Design review of the part built by this model. Coordinates are the model's own, in mm. A direction names the side the tool comes from. Coordinates: 2 decimals unless noted, no trailing zeros. Loops run counter-clockwise (first coordinate to the right, second up) from the corner with the lowest first, then second, coordinate; pieces in that order, holes last. Notation, with made-up numbers: (81.25, -20.5) -> (89.25, -20.5) arc R24 cw to (89.25, 1.5) -> close; hole circle Ø10 at (59, 26.25). An arc over 180 degrees is marked (long way). One line per item, written item: value. Start each with the question number.
1. Add section C-C on x = 22.5. Write out the cut boundary in (y, z), plus the area to 3 significant figures.
2. Add section B-B on z = 24.5. Write out the cut boundary in (x, y), plus the area to 3 significant figures.
3. Add section D-D on y = 19.5. Write out the cut boundary in (x, z).
4. Add section A-A on y = 34. Write out the cut boundary in (x, z), plus the area to 3 significant figures.
5. For probe 1 along X at (y, z) = (19, 21); probe 2 along Y at (x, z) = (23, 30); probe 3 along Y at (x, z) = (23, 28), list the stretches that pass through material, from the lowest coordinate up.
6. Machinability: for faces 1 (the flat face through (6, 35, 0)), 2 (the flat face through (0, 15, 16)), 3 (the flat face through (12.7, 15, 16)), which of the approach directions +Z, -Z, +X, -X, +Y, -Y give a long, thin tool a straight path to every point of the face, cutting with its end or side? Answer none if there is none.
7. Insertion check: pin 1 (3 mm diameter, centred on x = -2, z = 25.5, fed in from -Y); pin 2 (9.5 mm diameter, centred on y = 18.5, z = 20, fed in from +X). Each pin has a flat end and moves straight along its axis. Give the tip position at first contact, or say it passes through.
```python
from build123d import *

# Parameters (mm, degrees)
F1_DEPTH = 31.75
F3_DEPTH = 12.7
F5_DEPTH = 12.7


with BuildPart() as f1:
    # F0 (on Top) → F1 (new body)
    with BuildSketch(Plane.XY):
        Polygon((0, 25.4), (0, 0), (12.7, 0), (12.7, 25.4), (25.4, 25.4), (25.4, 57.15), (-12.7, 57.15), (-12.7, 25.4), align=None)
    extrude(amount=F1_DEPTH)

    # F2 (on face) → F3 (cut)
    with BuildSketch(Plane(origin=(-12.7, 0, 0), x_dir=(0, -1, 0), z_dir=(-1, 0, 0))):
        Polygon((-38.1, 31.75), (-25.4, 0), (-25.4, 31.75), align=None)
    extrude(amount=-F3_DEPTH, mode=Mode.SUBTRACT)

    # F4 (on face) → F5 (cut)
    with BuildSketch(Plane.YZ.offset(25.4)):
        Polygon((25.4, 0), (38.1, 31.75), (25.4, 31.75), align=None)
    extrude(amount=-F5_DEPTH, mode=Mode.SUBTRACT)


solid = f1.part
```
Worked answers:
1. outline: (25.4, 0) -> (57.15, 0) -> (57.15, 31.75) -> (38.1, 31.75) -> close
1. area: 806 mm²
2. outline: (-12.7, 35.2) -> (0, 35.2) -> (0, 0) -> (12.7, 0) -> (12.7, 35.2) -> (25.4, 35.2) -> (25.4, 57.15) -> (-12.7, 57.15) -> close
2. area: 1,280 mm²
3. outline: (0, 0) -> (12.7, 0) -> (12.7, 31.75) -> (0, 31.75) -> close
4. outline: (-12.7, 0) -> (25.4, 0) -> (25.4, 21.5) -> (12.7, 21.5) -> (12.7, 31.75) -> (0, 31.75) -> (0, 21.5) -> (-12.7, 21.5) -> close
4. area: 949 mm²
5. probe 1: x = 0 to 12.7
5. probe 2: y = 37.4 to 57.15
5. probe 3: y = 36.6 to 57.15
6. face 1: -Z, +X, -X, +Y, -Y
6. face 2: +Z, -X, -Y
6. face 3: +Z, +X, -Y
7. pin 1: stops at y = 35
7. pin 2: stops at x = 12.7
